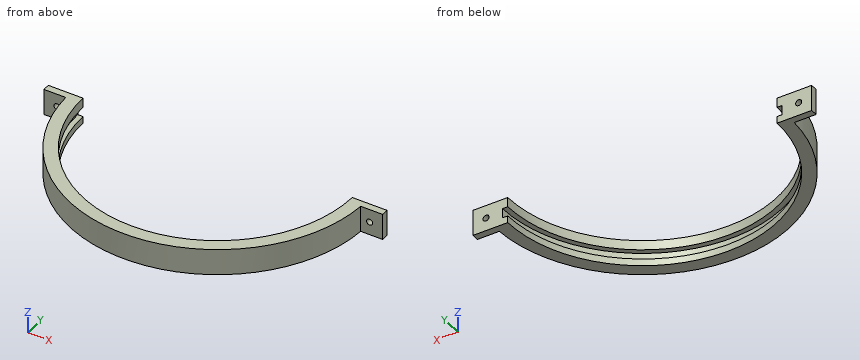
Autodesk Fusion 360 part; units mm, degrees
sketch "Sketch1" plane through (0, 0, 0) normal (0, 0, 1) x (1, 0, 0)
  circle A0 centre (0, 0) radius 87.5
  circle A1 centre (0, 0) radius 77.5
  line L0 (77.5, 0) -> (97.5, 0)
  line L1 (97.5, 0) -> (97.5, -97.5)
  line L2 (97.5, -97.5) -> (77.5, -97.5)
  line L3 (77.5, -97.5) -> (77.5, 0)
  line L4 (-77.5, 0) -> (-97.5, 0)
  line L5 (-97.5, 0) -> (-97.5, -97.5)
  line L6 (-97.5, -97.5) -> (-77.5, -97.5)
  line L7 (-77.5, -97.5) -> (-77.5, 0)
  line L8 (97.5, -97.5) -> (-97.5, -97.5)
  line L9 (-97.5, -97.5) -> (-97.5, -102.5)
  line L10 (-97.5, -102.5) -> (97.5, -102.5)
  line L11 (97.5, -102.5) -> (97.5, -97.5)
  dimension "d1" = 155
  dimension "d2" = 175
  dimension "d15" = 97.5
  dimension "d16" = 5
  dimension "d17" = 10
  dimension "d18" = 20
  dimension "d19" = 20
extrude "Extrude1" add sketch "Sketch1" along normal blind 15 contours A0 L0 L1 L2 L3 L8 | A0 L0 L3 | A0 L4 L7 | A0 L4 L5 L6 L7 L8 | A0 L3 L7 L8 | A0 A1 L3 L7 | L2 L6 L8 L9 L10 L11
sketch "Sketch2" plane through (0, 0, 0) normal (0, 0, 1) x (1, 0, 0)
  circle A0 centre (0, 0) radius 80.5
  dimension "d10" = 161
extrude "Extrude2" cut sketch "Sketch2" along normal blind 5.5 from surface at 4
sketch "Sketch3" plane through (0, 0, 15) normal (0, 0, 1) x (-1, 0, 0)
  line L0 (77.5, 0) -> (97.5, 0)
  line L1 (97.5, 0) -> (97.5, 102.5)
  line L2 (97.5, 102.5) -> (-97.5, 102.5)
  line L3 (-97.5, 102.5) -> (-97.5, 0)
  line L4 (-97.5, 0) -> (-77.5, 0)
  arc A0 (77.5, 0) -> (-77.5, 0) centre (0, 0) ccw
  line L5 (-30, 102.5) -> (30, 102.5)
  line L6 (30, 102.5) -> (30, 97.5)
  line L7 (30, 97.5) -> (-30, 97.5)
  line L8 (-30, 97.5) -> (-30, 102.5)
  dimension "d22" = 30
  dimension "d23" = 30
extrude "Extrude3" add sketch "Sketch3" along normal blind 30 contours L2 L5 L6 L7 L8
fillet "Fillet2" radius 15 4 edges at (-30, -100, 45) (30, -100, 45) (-30, -100, 15) (30, -100, 15)
sketch "Sketch4" plane through (0, -97.5, 0) normal (0, 1, 0) x (-1, 0, 0)
  arc A0 (-15, 45) -> (-30, 30) centre (-15, 30) ccw
  arc A1 (-45, 15) -> (-30, 30) centre (-45, 30) ccw
  line L0 (-45, 15) -> (45, 15)
  arc A2 (30, 30) -> (45, 15) centre (45, 30) ccw
  arc A3 (30, 30) -> (15, 45) centre (15, 30) ccw
  line L1 (15, 45) -> (-15, 45)
  line L2 (-97.5, 7.5) -> (97.5, 7.5) construction
  line L3 (-45, 0) -> (45, 0)
  line L4 (15, -30) -> (-15, -30)
  arc A4 (15, -30) -> (30, -15) centre (15, -15) ccw
  arc A5 (45, 0) -> (30, -15) centre (45, -15) ccw
  arc A6 (-30, -15) -> (-15, -30) centre (-15, -15) ccw
  arc A7 (-30, -15) -> (-45, 0) centre (-45, -15) ccw
  point P0 (0, 30)
  point P1 (-97.5, 7.5)
  point P2 (97.5, 7.5)
  point P3 (0, -15)
  dimension "d28" = 15
sketch "Sketch5" plane through (0, 0, 0) normal (0, 0, -1) x (1, 0, 0)
  line L0 (-97.5, 0) -> (-77.5, 0)
  arc A0 (77.5, 0) -> (-77.5, 0) centre (0, 0) ccw
  line L1 (77.5, 0) -> (97.5, 0)
  line L2 (97.5, 0) -> (97.5, 102.5)
  line L3 (97.5, 102.5) -> (-97.5, 102.5)
  line L4 (-97.5, 102.5) -> (-97.5, 0)
  line L5 (80, 102.5) -> (-80, 102.5)
  line L6 (-80, 102.5) -> (-80, 97.5)
  line L7 (-80, 97.5) -> (80, 97.5)
  line L8 (80, 97.5) -> (80, 102.5)
  dimension "d39" = 80
  dimension "d40" = 80
extrude "Extrude4" add sketch "Sketch5" along normal blind 30 contours L3 L5 L6 L7 L8
fillet "Fillet4" radius 15 4 edges at (80, -100, -30) (-80, -100, -30) (-80, -100, 0) (80, -100, 0)
sketch "Sketch6" plane through (0, -97.5, 0) normal (0, 1, 0) x (-1, 0, 0)
  arc A0 (65, -30) -> (80, -15) centre (65, -15) ccw
  arc A1 (95, 0) -> (80, -15) centre (95, -15) ccw
  line L0 (95, 0) -> (-95, 0)
  arc A2 (-80, -15) -> (-95, 0) centre (-95, -15) ccw
  arc A3 (-80, -15) -> (-65, -30) centre (-65, -15) ccw
  line L1 (-65, -30) -> (65, -30)
  line L2 (-77.5, 15) -> (77.5, 15)
  point P0 (0, -15)
  point P1 (0, 30)
  point P2 (50, -15)
  point P3 (-50, -15)
  dimension "d49" = 15
  dimension "d50" = 15
  dimension "d53" = 50
  dimension "d54" = 50
hole "Hole2" at (0, -97.5, -15) at (0, -97.5, 30) at (-50, -97.5, -15) at (50, -97.5, -15) direction (0, -1, 0) diameter 4 end through all
sketch "Sketch7" plane through (0, 0, 0) normal (0, 1, 0) x (-1, 0, 0)
  line L0 (77.5, 9.5) -> (80.5, 9.5)
  line L1 (80.5, 9.5) -> (80.5, 4)
  line L2 (80.5, 4) -> (77.5, 4)
  line L3 (77.5, 4) -> (77.5, 0)
  line L4 (77.5, 0) -> (97.5, 0)
  line L5 (97.5, 0) -> (97.5, 15)
  line L6 (97.5, 15) -> (77.5, 15)
  line L7 (77.5, 15) -> (77.5, 9.5)
  line L8 (-77.5, 0) -> (-97.5, 0)
  line L9 (-97.5, 0) -> (-97.5, 15)
  point P0 (90, 7.5)
  point P1 (-90, 7.5)
  dimension "d55" = 7.5
  dimension "d56" = 7.5
  dimension "d57" = 7.5
  dimension "d58" = 7.5
hole "Hole3" at (-90, 0, 7.5) at (90, 0, 7.5) direction (0, -1, 0) diameter 3.5 depth 15 tip angle 180
fillet "Fillet5" radius 10 2 edges at (0, -97.5, 0) (0, -97.5, 15)
sketch "Sketch8" plane through (0, 0, 0) normal (0, 0, -1) x (1, 0, 0)
  line L0 (-95, 87.5) -> (-95, 102.5)
  line L1 (-95, 102.5) -> (-97.5, 102.5)
  line L2 (-97.5, 102.5) -> (-97.5, 0)
  line L3 (-97.5, 0) -> (-77.5, 0)
  arc A0 (77.5, 0) -> (-77.5, 0) centre (0, 0) ccw
  line L4 (77.5, 0) -> (97.5, 0)
  line L5 (97.5, 0) -> (97.5, 102.5)
  line L6 (97.5, 102.5) -> (95, 102.5)
  line L7 (95, 102.5) -> (95, 87.5)
  line L8 (95, 87.5) -> (-95, 87.5)
  circle A1 centre (0, 0) radius 85
  line L9 (97.5, 0) -> (84.9058, 0)
  line L10 (84.9058, 0) -> (84.9058, 4)
  line L11 (84.9058, 4) -> (97.5, 4)
  line L12 (97.5, 4) -> (97.5, 0)
  line L13 (-97.5, 0) -> (-84.9058, 0)
  line L14 (-84.9058, 0) -> (-84.9058, 4)
  line L15 (-84.9058, 4) -> (-97.5, 4)
  line L16 (-97.5, 4) -> (-97.5, 0)
  line L17 (-97.5, 4) -> (97.5, 4)
  line L18 (97.5, 4) -> (97.5, 102.5)
  line L19 (97.5, 102.5) -> (-97.5, 102.5)
  line L20 (-97.5, 102.5) -> (-97.5, 4)
  dimension "d64" = 170
  dimension "d65" = 4
  dimension "d66" = 4
extrude "Extrude5" cut sketch "Sketch8" along normal through all and the other way through all contours L0 L1 L2 L5 L6 L7 L8 A1 L11 L15 L17 L18 L19 L20 | L0 L7 L8 L19
equation "d15 = d2 / 2 + 10 mm"
equation "d18 = d17 + 10 mm"
equation "d19 = d18"
equation "d23 = d22"
equation "d40 = d39"
equation "d56 = d55"
equation "d58 = d57"
equation "d66 = d65"
Build history of the part. All positions in model axes, mm. Give positions to 0.01 mm unless a question says otherwise; leave off trailing zeros. Loops run counter-clockwise (first coordinate to the right, second up) from the corner with the lowest first, then second, coordinate; pieces in that order, holes last.
Item 1: Slice it at D-D, the plane y = -18. List the corners of the cut face in (x, z), and give its area (3 significant figures).
Answers follow:
outline: (-83.07, 0) - (-75.38, 0) - (-75.38, 4) - (-78.46, 4) - (-78.46, 9.5) - (-75.38, 9.5) - (-75.38, 15) - (-83.07, 15) - close; (75.38, 0) - (83.07, 0) - (83.07, 15) - (75.38, 15) - (75.38, 9.5) - (78.46, 9.5) - (78.46, 4) - (75.38, 4) - close
area: 197 mm2
Item 2: Slice it at A-A, the plane x = -90. List the corners of the cut face in (y, z), and give its area (3 significant figures).
Answers follow:
outline: (-4, 0) - (0, 0) - (0, 5.75) - (-4, 5.75) - close; (-4, 9.25) - (0, 9.25) - (0, 15) - (-4, 15) - close
area: 46.0 mm2
Item 3: Slice it at C-C, the plane x = 0. List the corners of the cut face in (y, z).
Answers follow:
outline: (-85, 0) - (-77.5, 0) - (-77.5, 4) - (-80.5, 4) - (-80.5, 9.5) - (-77.5, 9.5) - (-77.5, 15) - (-85, 15) - close
Item 4: Flat gauge pins, fed straight in: pin 1 (3 mm diameter, centred on y = -71, z = 4.5, fed in from -X); pin 2 (6.5 mm diameter, centred on x = -90.5, z = 4, fed in from -Y); pin 3 (4 mm diameter, centred on y = -13.5, z = 6, fed in from +X); pin 4 (3 mm diameter, centred on x = -90, z = 7.5, fed in from -Y). Where does each tip first touch, or does it go through?
Answers follow:
pin 1: stops at x = -48.94
pin 2: stops at y = -4
pin 3: stops at x = 84.22
pin 4: passes through
Item 5: Drill centre lines: line 1 (X direction, y = -2.25, z = 7.5); line 2 (Z direction, x = 90, y = -3.1); line 3 (X direction, y = -2.85, z = 7.5). Where is each one in solid material? Low to high.
Answers follow:
line 1: x = -97.5 to -91.75, -88.25 to -80.47, 80.47 to 88.25, 91.75 to 97.5
line 2: z = 0 to 5.75, 9.25 to 15
line 3: x = -97.5 to -91.75, -88.25 to -80.45, 80.45 to 88.25, 91.75 to 97.5
